Work out the finished part from the listing and answer in its coordinate system (mm). Face numbers are marked on the shaded views. A direction names the side the tool comes from. Give positions to 0.01 mm unless a question says otherwise; leave off trailing zeros. Loops run counter-clockwise (first coordinate to the right, second up) from the corner with the lowest first, then second, coordinate; pieces in that order, holes last. Notation, with made-up numbers: M 21.25,-17 L 58.25,-17 A32 cw 58.25,18 Z; hole C -11.75,43.25 d1. An arc over 180 degrees is marked long. Answer as a JSON object with one key per item and string values. Group by question number.
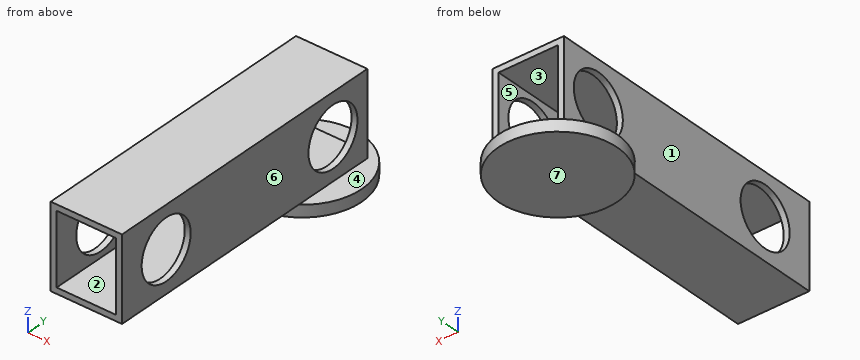
```python
from build123d import *

# Parameters (mm, degrees)
SKETCH_1_R          = 50
EXTRUDE_1_DEPTH     = 10
SKETCH_3_W          = 60
SKETCH_3_H          = 60
EXTRUDE_2_DEPTH     = 70
SKETCH_4_W          = 60
SKETCH_4_H          = 70
EXTRUDE_3_DEPTH     = 190
SKETCH_5_R          = 25
CUT_EXTRUDE_4_DEPTH = 190
SKETCH_6_W          = 50
SKETCH_6_H          = 60
CUT_EXTRUDE_5_DEPTH = 287.006992922


with BuildPart() as part:
    # 草图1 → 凸台-拉伸1 (new body)
    with BuildSketch(Plane.XY):
        Circle(SKETCH_1_R)
    extrude(amount=EXTRUDE_1_DEPTH)

    # 草图3 → 凸台-拉伸2 (add)
    with BuildSketch(Plane.XY.offset(10)):
        Rectangle(SKETCH_3_W, SKETCH_3_H)
    extrude(amount=EXTRUDE_2_DEPTH)

    # 草图4 → 凸台-拉伸3 (add)
    with BuildSketch(Plane.XZ.offset(30)):
        with Locations((0, 45)):
            Rectangle(SKETCH_4_W, SKETCH_4_H)
    extrude(amount=EXTRUDE_3_DEPTH)

    # 草图5 → 切除-拉伸4 (cut)
    with BuildSketch(Plane.ZY.offset(30)):
        with Locations(Location((45, -5, 0), (0, 0, 270))):
            Circle(SKETCH_5_R)
        with Locations(Location((45, -175, 0), (0, 0, 270))):
            Circle(SKETCH_5_R)
    extrude(amount=-CUT_EXTRUDE_4_DEPTH, mode=Mode.SUBTRACT)

    # 草图6 → 切除-拉伸5 (cut, through all)
    with BuildSketch(Plane.XZ.offset(220)):
        with Locations((0, 45)):
            Rectangle(SKETCH_6_W, SKETCH_6_H)
    extrude(amount=-CUT_EXTRUDE_5_DEPTH, mode=Mode.SUBTRACT)


solid = part.part
```
Item 1: A tool of negligible diameter and unlimited length cuts with its end or side. For the marked faces 5, 6 and 7, from which of +Z, -Z, +X, -X, +Y, -Y can it reach the whole face along a straight path? Write none if from no direction.
Item 2: A cutting plane is placed at C-C (z = 39). Determine the outline of the cut face in (x, y).
Item 3: A cutting plane is placed at A-A (x = 0). Determine the outline of the cut face in (y, z).
Item 4: Given pin 1 Ø25 at (x, y) = (9.5, -134.5) entering from -Z; pin 2 Ø12 at (x, z) = (31.5, 41) entering from +Y; pin 3 Ø8 at (y, z) = (-113, 68) entering from +X, each flat-ended and moving along its own axis, determine where each tip first touches the part or whether it passes through.
Item 5: A cutting plane is placed at D-D (y = -203.5). Determine the outline of the cut face in (x, z), and give its area (3 significant figures).
Item 6: A cutting plane is placed at B-B (y = -175). Determine the outline of the cut face in (x, z), and give its area (3 significant figures).
Item 7: For a pull along X with two mould halves and no side action, classify the marked faces 1, 2, 3 and 4 as pulls with the +X half, pulls with the -X half, needs draft (parallel to the pull), parting line crosses it, or undercut.
Item 8: Find the intervals of material crossed by probe 1 along Z at (x, y) = (-7, -106); probe 2 along Z at (x, y) = (-28.6, -5); probe 3 along X at (y, z) = (21, 16.5), in increasing order. Write a range as [from, to].
The answers:
{
 "1": {"face 5": "+Y, -Y", "face 6": "+Z, +X, +Y, -Y", "face 7": "-Z, +X, -X, +Y, -Y"},
 "2": {"outline": "M -30,-220 L -25,-220 L -25,-199.27 L -30,-199.27 Z; M -30,-150.73 L -25,-150.73 L -25,-29.27 L -30,-29.27 Z; M -30,19.27 L -25,19.27 L -25,30 L -30,30 Z; M 25,-220 L 30,-220 L 30,-199.27 L 25,-199.27 Z; M 25,-150.73 L 30,-150.73 L 30,-29.27 L 25,-29.27 Z; M 25,19.27 L 30,19.27 L 30,30 L 25,30 Z"},
 "3": {"outline": "M -220,10 L -50,10 L -50,0 L 50,0 L 50,10 L 30,10 L 30,15 L -220,15 Z; M -220,75 L 30,75 L 30,80 L -220,80 Z"},
 "4": {"pin 1": "stops at z = 10", "pin 2": "stops at y = 30", "pin 3": "stops at x = 30"},
 "5": {"outline": "M -30,10 L 30,10 L 30,80 L -30,80 Z; hole M -25,15 L 25,15 L 25,75 L -25,75 Z", "area": "1,200 mm^2"},
 "6": {"outline": "M -30,10 L 30,10 L 30,20 L 25,20 L 25,15 L -25,15 L -25,20 L -30,20 Z; M -30,70 L -25,70 L -25,75 L 25,75 L 25,70 L 30,70 L 30,80 L -30,80 Z", "area": "700 mm^2"},
 "7": {"face 1": "pulls with the -X half", "face 2": "undercut", "face 3": "undercut", "face 4": "needs draft"},
 "8": {"probe 1": "z = [10, 15], [75, 80]", "probe 2": "z = [0, 20], [70, 80]", "probe 3": "x = [-30, -25], [25, 30]"}
}
